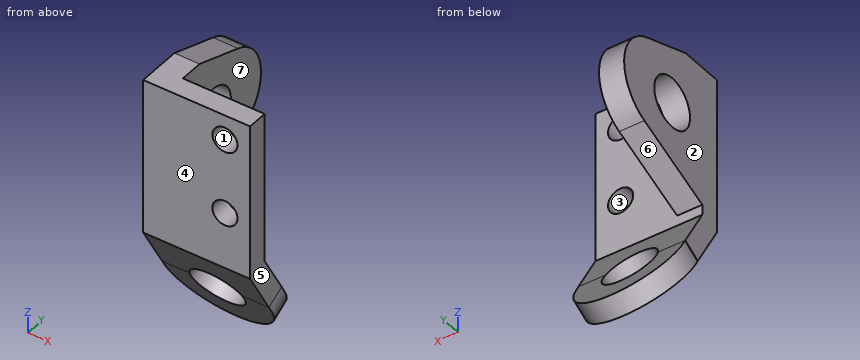
```python
from build123d import *

# Parameters (mm, degrees)
EXTRUDE_1_DEPTH     = 34
CUT_EXTRUDE_1_REACH = 72.355
SKETCH_2_R          = 4
EXTRUDE_2_DEPTH     = 8
CUT_EXTRUDE_2_REACH = 78.907
SKETCH_4_R          = 8
CUT_EXTRUDE_3_REACH = 80.3
SKETCH_6_R          = 8.5
CUT_EXTRUDE_4_REACH = 78.907
SKETCH_9_R          = 17
EXTRUDE_5_DEPTH     = 6.5
CUT_EXTRUDE_6_REACH = 81.317
SKETCH_13_R         = 8.5


with BuildPart() as part:
    # 草图1 → 凸台-拉伸1 (new body)
    with BuildSketch(Plane(origin=(0, 0, 0), x_dir=(0, 0, -1), z_dir=(1, 0, 0))):
        Polygon((0, 0), (28.258330249, 0), (56.194863729, 16.129165125), (59.444863729, 10.5), (30, -6.5), (-20, -6.5), (-20, 0), align=None)
    extrude(amount=-EXTRUDE_1_DEPTH)

    # 草图2 → 切除-拉伸1 (cut, up to next)
    with BuildSketch(Plane(origin=(0, 0, 0), x_dir=(1, 0, 0), z_dir=(0, 1, 0)), mode=Mode.PRIVATE) as cut_extrude_1_sk1:
        with Locations(Location((-8, -12, 0), (0, 0, 270))):
            Circle(SKETCH_2_R)
    cut_extrude_1_tool1 = extrude(cut_extrude_1_sk1.sketch, amount=-CUT_EXTRUDE_1_REACH, mode=Mode.PRIVATE) & part.part
    # 草图2 → 切除-拉伸1 (cut, up to next)
    with BuildSketch(Plane(origin=(0, 0, 0), x_dir=(1, 0, 0), z_dir=(0, 1, 0)), mode=Mode.PRIVATE) as cut_extrude_1_sk2:
        with Locations(Location((-8, 12, 0), (0, 0, 270))):
            Circle(SKETCH_2_R)
    cut_extrude_1_tool2 = extrude(cut_extrude_1_sk2.sketch, amount=-CUT_EXTRUDE_1_REACH, mode=Mode.PRIVATE) & part.part
    add(cut_extrude_1_tool1.solids().sort_by_distance((-8, 0, 12))[0], mode=Mode.SUBTRACT)
    add(cut_extrude_1_tool2.solids().sort_by_distance((-8, 0, -12))[0], mode=Mode.SUBTRACT)

    # 草图3 → 凸台-拉伸2 (add)
    with BuildSketch(Plane.ZY.offset(34)):
        with BuildLine():
            Line((-25, 0), (-13.76612817, 25.957660212))
            ThreePointArc((-13.76612817, 25.957660212), (0.641385669, 34.986281207), (14.224811704, 24.759698727))
            Line((14.224811704, 24.759698727), (20, 7.5))
            Line((20, 7.5), (20, 0))
            Line((20, 0), (-25, 0))
        make_face()
    extrude(amount=-EXTRUDE_2_DEPTH)

    # 草图4 → 切除-拉伸2 (cut, up to next)
    with BuildSketch(Plane.ZY.offset(34), mode=Mode.PRIVATE) as cut_extrude_2_sk1:
        with Locations((0, 13.5)):
            Circle(SKETCH_4_R)
    cut_extrude_2_tool1 = extrude(cut_extrude_2_sk1.sketch, amount=-CUT_EXTRUDE_2_REACH, mode=Mode.PRIVATE) & part.part
    add(cut_extrude_2_tool1.solids().sort_by_distance((-34, 13.5, 0))[0], mode=Mode.SUBTRACT)

    # 草图6 → 切除-拉伸3 (cut, up to next)
    with BuildSketch(Plane(origin=(0, -12.236215932, -7.064582562), x_dir=(1, 0, 0), z_dir=(0, 0.8660254037844378, 0.5000000000000017)), mode=Mode.PRIVATE) as cut_extrude_3_sk1:
        with Locations(Location((-17, 41.472431864, 0), (0, 0, 270))):
            Circle(SKETCH_6_R)
    cut_extrude_3_tool1 = extrude(cut_extrude_3_sk1.sketch, amount=-CUT_EXTRUDE_3_REACH, mode=Mode.PRIVATE) & part.part
    add(cut_extrude_3_tool1.solids().sort_by_distance((-17, 8.5, -42.980762))[0], mode=Mode.SUBTRACT)

    # 草图8 → 切除-拉伸4 (cut, up to next)
    with BuildSketch(Plane(origin=(0, 0, 0), x_dir=(0, 0, -1), z_dir=(1, 0, 0)), mode=Mode.PRIVATE) as cut_extrude_4_sk1:
        Polygon((44.722431864, 2), (41.472431864, 7.629165125), (56.194863729, 16.129165125), (59.444863729, 10.5), align=None)
    cut_extrude_4_tool1 = extrude(cut_extrude_4_sk1.sketch, amount=-CUT_EXTRUDE_4_REACH, mode=Mode.PRIVATE) & part.part
    add(cut_extrude_4_tool1.solids().sort_by_distance((0, 9.064583, -50.458648))[0], mode=Mode.SUBTRACT)

    # 草图9 → 凸台-拉伸5 (add)
    with BuildSketch(Plane(origin=(0, -12.236215932, -7.064582562), x_dir=(1, 0, 0), z_dir=(0, 0.8660254037844378, 0.5000000000000017))):
        with Locations((-17, 41.472431864)):
            Circle(SKETCH_9_R)
    extrude(amount=-EXTRUDE_5_DEPTH)

    # 草图13 → 切除-拉伸6 (cut, up to next)
    with BuildSketch(Plane(origin=(0, -12.236215932, -7.064582562), x_dir=(1, 0, 0), z_dir=(0, 0.8660254037844378, 0.5000000000000017)), mode=Mode.PRIVATE) as cut_extrude_6_sk1:
        with Locations(Location((-17, 41.472431864, 0), (0, 0, 270))):
            Circle(SKETCH_13_R)
    cut_extrude_6_tool1 = extrude(cut_extrude_6_sk1.sketch, amount=-CUT_EXTRUDE_6_REACH, mode=Mode.PRIVATE) & part.part
    add(cut_extrude_6_tool1.solids().sort_by_distance((-17, 8.5, -42.980762))[0], mode=Mode.SUBTRACT)


solid = part.part
```
Here's how the part is built. I have some questions about the finished solid (model axes, mm). Face numbers are marked on the shaded views. A direction names the side the tool comes from. Coordinates: 2 decimals unless noted, no trailing zeros. Order: outer loops, then holes, each group sorted by start corner. A loop starts at its lowest first (then second) coordinate and runs counter-clockwise, first axis right, second up.
Item 1: Which directions (+Z, -Z, +X, -X, +Y, -Y) give clear straight access to the entire face, cutting with the end or side of a thin tool? Please do the marked faces 5, 6 and 7.
Response values:
face 5: +Z, -Z, +X, +Y, -Y
face 6: +X, -X, +Y
face 7: +Z, +X, +Y
Item 2: If we section it at B-B, the plane x = -20: List the corners of the cut face in (y, z) for me.
Response values:
outline: (-6.5, -30) - (-1.11, -39.34) - (4.52, -36.09) - (0, -28.26) - (0, 20) - (-6.5, 20) - close; (6.85, -53.12) - (11.24, -60.72) - (16.87, -57.47) - (12.48, -49.87) - close
Item 3: I need wall thicknesses on probe 1 along Y at (x, z) = (-29.5, 0); probe 2 along Z at (x, y) = (-29, 13) (3 decimals); probe 3 along X at (y, z) = (-5, -12). Which ranges of each line are inside material? Lowest first, please.
Response values:
probe 1: y = -6.5 to 5.5, 21.5 to 35
probe 2: z = -54.287 to -50.775, -19.374 to -7.984, 7.984 to 18.16
probe 3: x = -34 to -12, -4 to 0
Item 4: Thinking about a two-plate mould opening in X: for the marked faces 1, 2, 3 and 4, which applies, pulls with the +X half, pulls with the -X half, needs draft (parallel to the pull), parting line crosses it, or undercut?
Response values:
face 1: undercut
face 2: pulls with the -X half
face 3: undercut
face 4: needs draft
Item 5: If we section it at D-D, the plane y = 9: Give the number of separate pieces and of enclosed holes in the cut face, then the cut area to 3 significant figures.
Response values:
separate pieces: 3
enclosed holes: 0
area: 504 mm2
Item 6: I'm going to push flat-ended pins straight in: pin 1 Ø1.5 at (x, z) = (-30.5, -50) entering from -Y; pin 2 Ø4 at (y, z) = (19, 1.5) entering from +X; pin 3 Ø2 at (x, y) = (-13, 12.5) entering from +Z; pin 4 Ø8 at (y, z) = (30.5, 5) entering from +X. Where does each tip first touch, or does it pass through?
Response values:
pin 1: stops at y = 4.61
pin 2: passes through
pin 3: stops at z = -49.02
pin 4: stops at x = -26
Item 7: If we section it at A-A, the plane z = -12: List the corners of the cut face in (x, y) for me.
Response values:
outline: (-34, -6.5) - (-12, -6.5) - (-12, 0) - (-26, 0) - (-26, 29) - (-34, 29) - close; (-4, -6.5) - (0, -6.5) - (0, 0) - (-4, 0) - close
Item 8: If we section it at C-C, the plane x = -31: List the corners of the cut face in (y, z) for me, then the cut area to 3 significant figures.
Response values:
outline: (-6.5, -30) - (7.69, -54.58) - (13.32, -51.33) - (0, -28.26) - (0, -25) - (25.96, -13.77) arc R15 ccw to (24.76, 14.22) - (7.5, 20) - (-6.5, 20) - close; hole circle Ø16 at (13.5, 0)
area: 1,440 mm2
